Verification items for this drawing (mm, ordinates from the low corner). A direction names the side the tool comes from. Coordinates: 2 decimals unless noted, no trailing zeros. Order: outer loops, then holes, each group sorted by start corner. A loop starts at its lowest first (then second) coordinate and runs counter-clockwise, first axis right, second up. Notation, with made-up numbers: M 6.5,-37.75 L 56.5,-37.75 A25 cw 56.5,-3.75 Z; hole C 64.25,40 d2. An arc over 180 degrees is marked long. Write item = value, one per line.
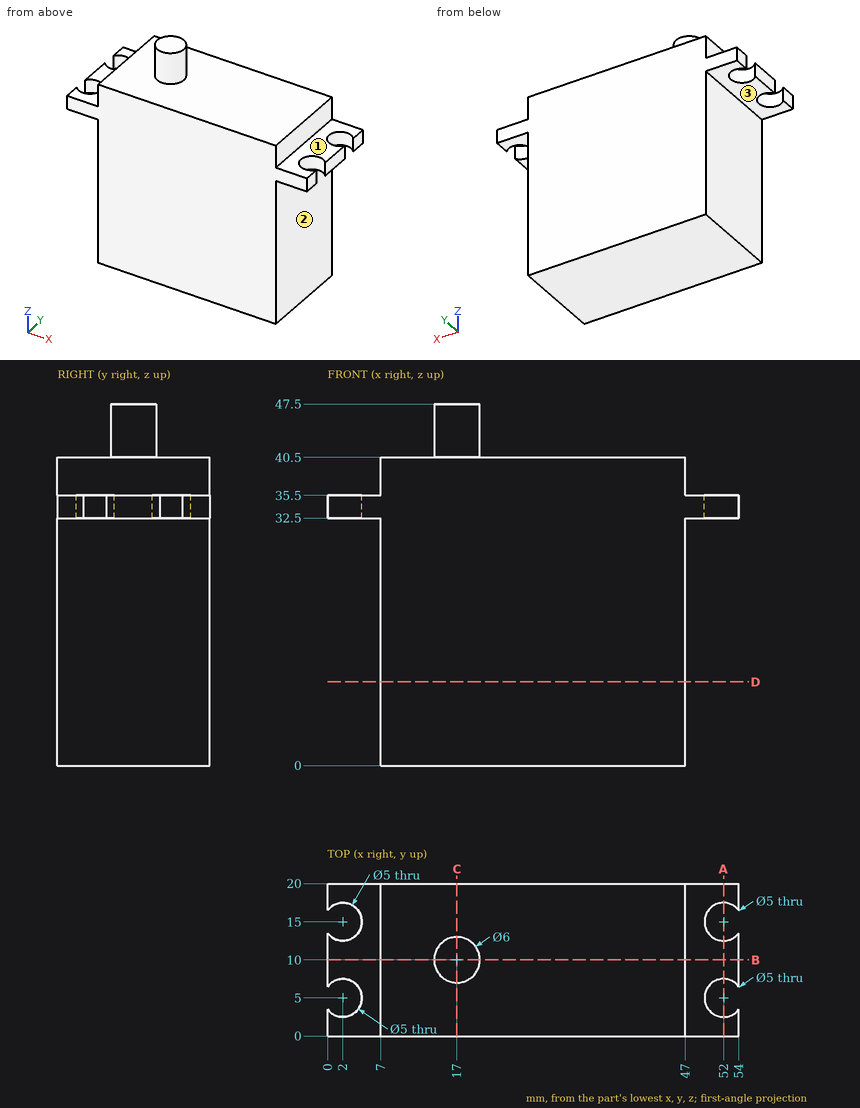
Item 1: Tool access check on the marked faces 1, 2 and 3. Record the directions out of +Z, -Z, +X, -X, +Y, -Y that give a thin tool (end or side, any length) a straight path to the whole face; none if there is none.
Report:
face_1 = +Z, +X, +Y, -Y
face_2 = -Z, +X, +Y, -Y
face_3 = -Z, -X, +Y, -Y
Item 2: Sectioned sample at A-A, the plane x = 52. Enter the section's corners in (y, z).
Report:
outline = M 0,32.5 L 2.5,32.5 L 2.5,35.5 L 0,35.5 Z; M 7.5,32.5 L 12.5,32.5 L 12.5,35.5 L 7.5,35.5 Z; M 17.5,32.5 L 20,32.5 L 20,35.5 L 17.5,35.5 Z
Item 3: Scan lines: L1, parallel to Y at x = 2, z = 33; L2, parallel to X at y = 8.5, z = 6.5; L3, parallel to Z at x = 45.5, y = 16.5. Record each from-to range of solid material in increasing order. Write a range as from..to.
Report:
L1 = 0..2.5, 7.5..12.5, 17.5..20
L2 = 7..47
L3 = 0..40.5
Item 4: Gauge pin test, flat ends, axial feed: pin 1 (3 mm diameter, centred on x = 2, y = 5, fed in from +Z); pin 2 (5.5 mm diameter, centred on y = 11.5, z = 37.5, fed in from -X); pin 3 (2 mm diameter, centred on x = 51.5, y = 13, fed in from -Z); pin 4 (2 mm diameter, centred on y = 13, z = 30.5, fed in from +X). Record the tip position at first contact, or that the pin passes through.
Report:
pin_1 = through
pin_2 = 0
pin_3 = 32.5
pin_4 = 47
Item 5: Sectioned sample at D-D, the plane z = 11. Enter the section's corners in (x, y).
Report:
outline = M 7,0 L 47,0 L 47,20 L 7,20 Z
Item 6: Sectioned sample at B-B, the plane y = 10. Enter the section's corners in (x, z).
Report:
outline = M 0,32.5 L 7,32.5 L 7,0 L 47,0 L 47,32.5 L 54,32.5 L 54,35.5 L 47,35.5 L 47,40.5 L 20,40.5 L 20,47.5 L 14,47.5 L 14,40.5 L 7,40.5 L 7,35.5 L 0,35.5 Z
Item 7: Sectioned sample at C-C, the plane x = 17. Enter the section's corners in (y, z).
Report:
outline = M 0,0 L 20,0 L 20,40.5 L 13,40.5 L 13,47.5 L 7,47.5 L 7,40.5 L 0,40.5 Z
